from build123d import *

# Parameters (mm, degrees)
F_4_40_TAPPED_HOLE1_D               = 2.2606
F_4_40_TAPPED_HOLE1_DEPTH           = 7.62
F_4_40_TAPPED_HOLE1_TIP             = 0.679152758
F_4_40_TAPPED_HOLE1_ON_FACE_2_D     = 2.2606
F_4_40_TAPPED_HOLE1_ON_FACE_2_DEPTH = 7.62
F_4_40_TAPPED_HOLE1_ON_FACE_2_TIP   = 0.679152758
F_4_40_TAPPED_HOLE1_ON_FACE_3_D     = 2.2606
F_4_40_TAPPED_HOLE1_ON_FACE_3_DEPTH = 7.62
F_4_40_TAPPED_HOLE1_ON_FACE_3_TIP   = 0.679152758
F_4_40_TAPPED_HOLE1_ON_FACE_4_D     = 2.2606
F_4_40_TAPPED_HOLE1_ON_FACE_4_DEPTH = 7.62
F_4_40_TAPPED_HOLE1_ON_FACE_4_TIP   = 0.679152758
SKETCH10_R                          = 20.50415
CUT_EXTRUDE3_DEPTH                  = 31.75
F_4_40_TAPPED_HOLE2_D               = 2.2606
F_4_40_TAPPED_HOLE2_DEPTH           = 7.62
F_4_40_TAPPED_HOLE2_TIP             = 0.679152758
CHAMFER1_SIZE                       = 1.27
SCALE1_SCALE                        = 2.362204724


# Read off the part's stored shape, not the designer's step: AdvancedHole3
with BuildPart() as part:
    # Sketch2 → Revolve1 (revolve)
    with BuildSketch(Plane(origin=(0, 0, 0), x_dir=(0, 0, -1), z_dir=(1, 0, 0))):
        Polygon((-18.542, 30.02915), (-12.192, 30.02915), (-12.192, 27.9781), (-8.5725, 27.9781), (-8.5725, 30.02915), (-6.0325, 30.02915), (-6.0325, 27.9781), (-2.413, 27.9781), (-2.413, 30.02915), (0, 30.02915), (0, 0), (-18.542, 0), align=None)
    revolve(axis=Axis((0, 0, 0), (0, 0, 1)))

    # #4-40 Tapped Hole1
    with Locations(Plane(origin=(0, -30.02915, 15.367), x_dir=(0, 0, -1), z_dir=(0, -1, 0))):
        with Locations((0, 0)):
            Hole(F_4_40_TAPPED_HOLE1_D / 2, depth=F_4_40_TAPPED_HOLE1_DEPTH)
            with Locations((0, 0, -(F_4_40_TAPPED_HOLE1_DEPTH + F_4_40_TAPPED_HOLE1_TIP / 2))):  # 118° drill point
                Cone(0, F_4_40_TAPPED_HOLE1_D / 2, F_4_40_TAPPED_HOLE1_TIP, mode=Mode.SUBTRACT)

    # #4-40 Tapped Hole1 on face 2
    with Locations(Plane(origin=(30.02915, 0, 15.367), x_dir=(0, 0, 1), z_dir=(1, 0, 0))):
        with Locations((0, 0)):
            Hole(F_4_40_TAPPED_HOLE1_ON_FACE_2_D / 2, depth=F_4_40_TAPPED_HOLE1_ON_FACE_2_DEPTH)
            with Locations((0, 0, -(F_4_40_TAPPED_HOLE1_ON_FACE_2_DEPTH + F_4_40_TAPPED_HOLE1_ON_FACE_2_TIP / 2))):  # 118° drill point
                Cone(0, F_4_40_TAPPED_HOLE1_ON_FACE_2_D / 2, F_4_40_TAPPED_HOLE1_ON_FACE_2_TIP, mode=Mode.SUBTRACT)

    # #4-40 Tapped Hole1 on face 3
    with Locations(Plane(origin=(-30.02915, 0, 15.367), x_dir=(0, 0, -1), z_dir=(-1, 0, 0))):
        with Locations((0, 0)):
            Hole(F_4_40_TAPPED_HOLE1_ON_FACE_3_D / 2, depth=F_4_40_TAPPED_HOLE1_ON_FACE_3_DEPTH)
            with Locations((0, 0, -(F_4_40_TAPPED_HOLE1_ON_FACE_3_DEPTH + F_4_40_TAPPED_HOLE1_ON_FACE_3_TIP / 2))):  # 118° drill point
                Cone(0, F_4_40_TAPPED_HOLE1_ON_FACE_3_D / 2, F_4_40_TAPPED_HOLE1_ON_FACE_3_TIP, mode=Mode.SUBTRACT)

    # #4-40 Tapped Hole1 on face 4
    with Locations(Plane(origin=(0, 30.02915, 15.367), x_dir=(0, 0, 1), z_dir=(0, 1, 0))):
        with Locations((0, 0)):
            Hole(F_4_40_TAPPED_HOLE1_ON_FACE_4_D / 2, depth=F_4_40_TAPPED_HOLE1_ON_FACE_4_DEPTH)
            with Locations((0, 0, -(F_4_40_TAPPED_HOLE1_ON_FACE_4_DEPTH + F_4_40_TAPPED_HOLE1_ON_FACE_4_TIP / 2))):  # 118° drill point
                Cone(0, F_4_40_TAPPED_HOLE1_ON_FACE_4_D / 2, F_4_40_TAPPED_HOLE1_ON_FACE_4_TIP, mode=Mode.SUBTRACT)

    # Sketch6 → Revolve2 (revolve)
    with BuildSketch(Plane(origin=(0, 0, 0), x_dir=(1, 0, 0), z_dir=(0, 1, 0)), mode=Mode.PRIVATE) as revolve2_sk:
        with BuildLine():
            Line((0, -18.542), (31.75, -18.542))
            ThreePointArc((31.75, -18.542), (22.450640303, -40.992640303), (0, -50.292))
            Line((0, -50.292), (0, -18.542))
        make_face()
    revolve(revolve2_sk.sketch.rotate(Axis((0, 0, 18.542), (0, 0, 1)), 90), axis=Axis((0, 0, 18.542), (0, 0, 1)))

    # Sketch10 → Cut-Extrude3 (cut)
    with BuildSketch(Plane(origin=(0, 0, 0), x_dir=(-1, 0, 0), z_dir=(0, 0, -1))):
        with Locations(Location((0, 0, 0), (0, 0, 90))):
            Circle(SKETCH10_R)
    extrude(amount=-CUT_EXTRUDE3_DEPTH, mode=Mode.SUBTRACT)

    # #4-40 Tapped Hole2
    with Locations(Plane(origin=(0, 0, 31.75), x_dir=(-1, 0, 0), z_dir=(0, 0, -1))):
        with Locations((0, 0)):
            Hole(F_4_40_TAPPED_HOLE2_D / 2, depth=F_4_40_TAPPED_HOLE2_DEPTH)
            with Locations((0, 0, -(F_4_40_TAPPED_HOLE2_DEPTH + F_4_40_TAPPED_HOLE2_TIP / 2))):  # 118° drill point
                Cone(0, F_4_40_TAPPED_HOLE2_D / 2, F_4_40_TAPPED_HOLE2_TIP, mode=Mode.SUBTRACT)

    # Chamfer1
    chamfer1_edges = [part.edges().sort_by_distance(p)[0] for p in [
        (0, -30.02915, 0),
    ]]
    chamfer(chamfer1_edges, length=CHAMFER1_SIZE)

    # AdvancedHole3 outline → AdvancedHole3 (revolve, cut)
    with BuildSketch(Plane.YX.offset(-36.83)):
        Polygon((3.81, 28.256858344), (0, 28.256858344), (0, 8.880183098), (2.5527, 10.414), (2.5527, 23.114), (3.81, 23.114), align=None)
    advancedhole3 = revolve(axis=Axis((0, 0, 36.83), (1, 0, 0)), mode=Mode.SUBTRACT)

    # Mirror2: AdvancedHole3 across plane
    add(advancedhole3.mirror(Plane(origin=(0, 0, 0), x_dir=(0, 0, 1), z_dir=(1, 0, 0))), mode=Mode.SUBTRACT)


with BuildPart() as part_1:
    # Scale1: scaled about (-5.1967e-05, 4.9002e-05, 24.526771352)
    add(part.part.scale(SCALE1_SCALE).moved(Location((7.079e-05, -6.6751e-05, -33.41048381))))


solid = part_1.part
Could you check a few things on this model? Use its own coordinates, in mm. A direction names the side the tool comes from. Give positions to 0.01 mm unless a question says otherwise; leave off trailing zeros. Answer in a Markdown table with one row per item. Add a question column.
Item 1: Please list where these lines run through material, in increasing order: probe 1 along Z at (x, y) = (-36, -59.5); probe 2 along Z at (x, y) = (-56, -35.5); probe 3 along Z at (x, y) = (0, 66).
Item 2: For faces 4 (the flat face through (-32, 58, -27.71)), 5 (the cylindrical face through (-61.81, -1.8, 0.92)), 6 (the flat face through (-44.8, -55.2, 10.39)), 7 (the cylindrical face through (61.81, 1.02, 0.42)), which set-ups out of +Z, -Z, +X, -X, +Y, -Y let a thin tool reach every point of the face, with its end or its side?
Item 3: I'm going to push flat-ended pins straight in: P1, Ø19.5, axis at y = 0, z = 53.59, coming from the +X side; P2, Ø8, axis at y = -30.5, z = 67, coming from the +X side; P3, Ø6, axis at x = 5, z = 31.5, coming from the +Y side. Where does each tip first touch, or does it pass through?
Item 4: We'd pull the mould along Z, two halves only. Please class faces 1 (the flat face through (-10, -1, 41.59)), 2 (the cylindrical face through (-0.6, -2.6, 50.7)), 3 (the cylindrical face through (64.518, -14.327, -8.945)): pulls with the +Z half, pulls with the -Z half, needs draft (parallel to the pull), parting line crosses it, or undercut.
Result:
| question | item | result |
|---|---|---|
| 1 | probe 1 | -31.8 to -27.71, -19.16 to -13.16, -4.61 to 38.47 |
| 1 | probe 2 | -33.41 to -27.71, -19.16 to -13.16, -4.61 to 45.44 |
| 1 | probe 3 | -33.41 to 0.22, 5.56 to 46.01 |
| 2 | face 4 | none |
| 2 | face 5 | -X |
| 2 | face 6 | -Z |
| 2 | face 7 | +X |
| 3 | P1 | x = 67.13 |
| 3 | P2 | x = 44.59 |
| 3 | P3 | y = 72.63 |
| 4 | face 1 | pulls with the -Z half |
| 4 | face 2 | needs draft |
| 4 | face 3 | undercut |
